Drawing for the job (mm, zero at the part's lowest x, y, z). A direction names the side the tool comes from. Round coordinates to 2 decimals unless told otherwise and drop trailing zeros. Write each loop counter-clockwise with the first axis right and the second up, starting at its lowest first coordinate (ties: lowest second). Pieces come first, ordered by that corner, then holes.
Item 1: 3-axis set-ups, long thin cutter, end or side, ignore diameter. For the marked faces 1 and 2: which of +Z, -Z, +X, -X, +Y, -Y reach the whole face in a straight line?
Item 2: Drop flat-ended pins along their axis: pin 1 Ø1.5 at (x, y) = (1.5, 1.5) entering from -Z; pin 2 Ø4 at (x, z) = (5, 5) entering from -Y; pin 3 Ø4 at (x, z) = (3.5, 10) entering from +Y. Give the stop position or say it passes through.
Item 3: Wall check: probe 1 along Z at (x, y) = (4, 6) (3 decimals); probe 2 along X at (y, z) = (9.5, 2); probe 3 along Z at (x, y) = (6.5, 8.5). Give the ranges that are in metal, low to high.
Item 4: Band-saw the part on A-A, the plane y = 6. Write the cut outline in (x, z) (3 decimals), then the cut area to 3 significant figures.
Item 5: Band-saw the part on D-D, the plane y = 1. Write the cut outline in (x, z), then the cut area to 3 significant figures.
Item 6: Band-saw the part on C-C, the plane x = 3.5. Write the cut outline in (y, z) (3 decimals), then the cut area to 3 significant figures.
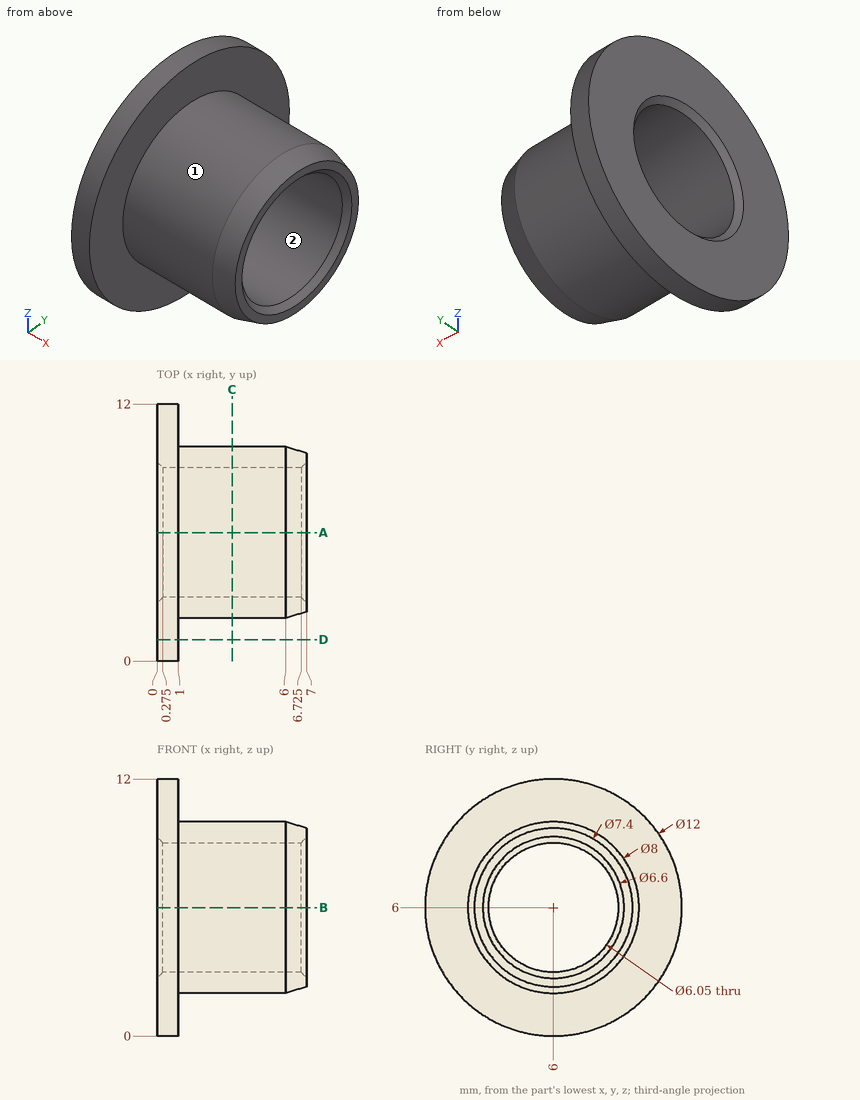
Results:
1. face 1: +X
1. face 2: +X, -X
2. pin 1: stops at z = 1.48
2. pin 2: stops at y = 2
2. pin 3: stops at y = 9.46
3. probe 1: z = 2 to 2.975, 9.025 to 10
3. probe 2: x = 0 to 1
3. probe 3: z = 3.07 to 4.3, 7.7 to 8.93
4. outline: (0, 0) - (1, 0) - (1, 2) - (6, 2) - (7, 2.3) - (7, 2.7) - (6.725, 2.975) - (0.275, 2.975) - (0, 2.7) - close; (0, 9.3) - (0.275, 9.025) - (6.725, 9.025) - (7, 9.3) - (7, 9.7) - (6, 10) - (1, 10) - (1, 12) - (0, 12) - close
4. area: 17.2 mm2
5. outline: (0, 2.68) - (1, 2.68) - (1, 9.32) - (0, 9.32) - close
5. area: 6.63 mm2
6. outline: circle Ø8 at (6, 6); hole circle Ø6.05 at (6, 6)
6. area: 21.5 mm2
